Can you work these out from the model? Positions are in its coordinate system, mm. A direction names the side the tool comes from. Give positions to 0.01 mm unless a question says otherwise; leave off trailing zeros. Order: outer loops, then holes, each group sorted by start corner. A loop starts at its lowest first (then second) coordinate and runs counter-clockwise, first axis right, second up. Notation, with made-up numbers: M 21.5,-20 L 64.5,-20 A10 cw 64.5,-2 Z; hole C 55,-3 d4. An arc over 180 degrees is marked long. Use one line per item in the form item = value. Start each with the question number.
1. I need wall thicknesses on L1, parallel to Z at x = -279, y = 325; L2, parallel to X at y = 314, z = 11; L3, parallel to Y at x = -262, z = 20.25. Which ranges of each line are inside material? Lowest first, please.
2. Will these pins go through, and if not, where does the flat tip stop? P1, Ø1.5, axis at x = -252.5, y = 309, coming from the +Z side; P2, Ø1, axis at x = -271, z = 13.5, coming from the +Y side; P3, Ø5, axis at y = 328, z = 12, coming from the -X side.
3. For faces 1 (the face through (-262.478, 313.576, 18.451)), 2 (the face through (-279.11, 328.53, 12.72)), which set-ups out of +Z, -Z, +X, -X, +Y, -Y let a thin tool reach every point of the face, with its end or its side?
4. I want a section at C-C, the plane x = -264.5. List the corners of the cut face in (y, z) for me.
5. I want a section at B-B, the plane z = 14.25. List the corners of the cut face in (x, y) for me, and give its area (3 significant figures).
6. I want a section at D-D, the plane z = 17.25. List the corners of the cut face in (x, y) for me.
7. I want a section at A-A, the plane y = 319. List the corners of the cut face in (x, z) for me.
```python
from build123d import *

# Parameters (mm, degrees)
VASTAGO_PROFILE_R = 3
GOMA_START        = 10.5
GOMA_DEPTH        = 4.5


with BuildPart() as part:
    # Vastago: sweep along a curve in space
    with BuildLine() as vastago_path:
        Line((-263.128358849, 316.504901668, 22), (-263.128358849, 316.504901668, 15))
    # Vastago profile (on start of the path) → Vastago (sweep)
    with BuildSketch(Plane(origin=(-263.128358849, 316.504901668, 22), x_dir=(-1, 0, 0), z_dir=(0, 0, -1))):
        Circle(VASTAGO_PROFILE_R)
    sweep(path=vastago_path.line)

    # Sk_Goma → Goma (add)
    with BuildSketch(Plane.XY.offset(GOMA_START)):
        Polygon((-249.511779913, 301.319751749), (-244.718766785, 307.724985949), (-276.744937786, 331.690051587), (-281.537950914, 325.284817387), align=None)
    extrude(amount=GOMA_DEPTH)


solid = part.part
```
Check result:
q1.L1 = 10.5 to 15
q1.L2 = -266.46 to -253.1
q1.L3 = 313.73 to 319.28
q2.P1 = 15
q2.P2 = 327.77
q2.P3 = -281.38
q3.face_1 = +Z
q3.face_2 = +Z, -Z, -X, +Y
q4.outline = M 312.54,10.5 L 322.53,10.5 L 322.53,15 L 319.17,15 L 319.17,22 L 313.84,22 L 313.84,15 L 312.54,15 Z
q5.outline = M -281.54,325.28 L -249.51,301.32 L -244.72,307.72 L -276.74,331.69 Z
q5.area = 320 mm2
q6.outline = C -263.13,316.5 d6
q7.outline = M -273.14,10.5 L -259.79,10.5 L -259.79,15 L -261.46,15 L -261.46,22 L -264.79,22 L -264.79,15 L -273.14,15 Z
